```python
from build123d import *

# Parameters (mm, degrees)
F0_W     = 431
F0_H     = 400
F1_DEPTH = 19
F2_R     = 12.5
F3_DEPTH = 12
F5_D     = 8
F5_DEPTH = 22
F5_TIP   = 2.4034424761


# Not quite as in the source:
# - a pattern or mirror of a feature is missing from the dataset's text; its kind, count and spacing are read off the source's solid


with BuildPart() as f1:
    # F0 (on Right) → F1 (new body)
    with BuildSketch(Plane.YZ):
        Rectangle(F0_W, F0_H)
    extrude(amount=F1_DEPTH)

    # F2 (on face) → F3 (cut)
    with BuildSketch(Plane(origin=(0, 0, 0), x_dir=(0, -1, 0), z_dir=(-1, 0, 0))):
        with Locations((-159.5, 166.5)):
            Circle(F2_R)
        with Locations((140.5, 166.5)):
            Circle(F2_R)
        with Locations((140.5, -166.5)):
            Circle(F2_R)
        with Locations((-159.5, -166.5)):
            Circle(F2_R)
    extrude(amount=-F3_DEPTH, mode=Mode.SUBTRACT)

    # F5
    with Locations(Plane.XY.offset(200)):
        with Locations((7, 159.5), (7, -140.5)):
            f5 = Hole(F5_D / 2, depth=F5_DEPTH)
            with Locations((0, 0, -(F5_DEPTH + F5_TIP / 2))):  # 118° drill point
                Cone(0, F5_D / 2, F5_TIP, mode=Mode.SUBTRACT)

    # F5_copies: F5 across plane
    add(f5.mirror(Plane(origin=(0, 0, 2.1e-05), x_dir=(-1, 0, 0), z_dir=(0, 0, -1))), mode=Mode.SUBTRACT)


solid = f1.part
```
Geometry: final body of the model. Coordinates: model frame, mm. A direction names the side the tool comes from. Coordinates: 2 decimals unless noted, no trailing zeros. Order: outer loops, then holes, each group sorted by start corner. A loop starts at its lowest first (then second) coordinate and runs counter-clockwise, first axis right, second up. Notation, with made-up numbers: (-36.75, 59) -> (-1.75, 59) arc R33 ccw to (-1.75, 91) -> close; hole circle Ø8 at (57, 19). An arc over 180 degrees is marked (long way). Write each question's results on one line, items separated by ' | '. Start each with the question number.
1) Material intervals for line 1 along Y through (x, z) = (7, 186); line 2 along Z through (x, y) = (2.5, 159.5); line 3 along Y through (x, z) = (5.25, -172), sorted ascending.
2) Mould query, pull axis Z, two halves, no side actions, for faces 1 (the flat face through (12, -140, -166)), 2 (the cylindrical face through (5.92, -146.27, 155.41)), 3 (the flat face through (9, -3, 200)), 4 (the flat face through (9, -3, -200)). Classes: released by +Z, released by -Z, zero draft, split by the parting line, or undercut.
3) Cut plane A-A, the plane z = -166.5. Output: boundary loops of the cut face in (x, y), and give its area (3 significant figures).
4) Cut plane B-B, the plane x = 7. Output: boundary loops of the cut face in (y, z).
5) First-contact query: pin 1 (20 mm diameter, centred on y = -140.5, z = 166.5, fed in from -X). Flat tip, straight axial feed; report the tip coordinate or a pass-through.
6) Set-up query: faces 5 (the flat face through (9, -215.5, -3)), 6 (the cylindrical face through (5.92, 153.73, 155.41)). Return all of +Z, -Z, +X, -X, +Y, -Y with unobstructed straight access to the full face (end or side cutting, diameter ignored); none if empty.
Checks:
1) line 1: -215.5 to -144.5, -136.5 to 155.5, 163.5 to 215.5 | line 2: -200 to -179, -154 to 154, 179 to 200 | line 3: -215.5 to -151.72, -129.28 to 148.28, 170.72 to 215.5
2) face 1: undercut | face 2: undercut | face 3: released by +Z | face 4: released by -Z
3) outline: (0, -215.5) -> (19, -215.5) -> (19, 215.5) -> (0, 215.5) -> (0, 172) -> (12, 172) -> (12, 147) -> (0, 147) -> (0, -128) -> (12, -128) -> (12, -153) -> (0, -153) -> close | area: 7,590 mm^2
4) outline: (-215.5, -200) -> (-144.5, -200) -> (-144.5, -178.34) arc R12.5 cw (long way) to (-136.5, -178.34) -> (-136.5, -200) -> (155.5, -200) -> (155.5, -178.34) arc R12.5 cw (long way) to (163.5, -178.34) -> (163.5, -200) -> (215.5, -200) -> (215.5, 200) -> (163.5, 200) -> (163.5, 178.34) arc R12.5 cw (long way) to (155.5, 178.34) -> (155.5, 200) -> (-136.5, 200) -> (-136.5, 178.34) arc R12.5 cw (long way) to (-144.5, 178.34) -> (-144.5, 200) -> (-215.5, 200) -> close
5) pin 1: x = 12
6) face 5: +Z, -Z, +X, -X, -Y | face 6: -X
